```python
from build123d import *

# Parameters (mm, degrees)
SZKIC1_W                                             = 60
SZKIC1_H                                             = 62
DODANIE_WYCI_GNI_CIE1_DEPTH                          = 12
SZKIC2_R                                             = 17
WYTNIJ_WYCI_GNI_CIE1_DEPTH                           = 337.608080711
POG_BIENIE_WALCOWE_POD_M5_WKR_T_DO_CZ_CI_D           = 5.5
POG_BIENIE_WALCOWE_POD_M5_WKR_T_DO_CZ_CI_CBORE_D     = 9
POG_BIENIE_WALCOWE_POD_M5_WKR_T_DO_CZ_CI_CBORE_DEPTH = 5
OTW_R_GWINTOWANY_M5X0_81_D                           = 4.2
SFAZOWANIE1_SIZE                                     = 5


with BuildPart() as part:
    # Szkic1 → Dodanie-wyciągnięcie1 (new body)
    with BuildSketch(Plane.XY):
        with Locations((30, 300)):
            Rectangle(SZKIC1_W, SZKIC1_H)
    extrude(amount=DODANIE_WYCI_GNI_CIE1_DEPTH)

    # Szkic2 → Wytnij-wyciągnięcie1 (cut, through all)
    with BuildSketch(Plane.XY.offset(12)):
        with Locations((31.5, 300)):
            Circle(SZKIC2_R)
    extrude(amount=-WYTNIJ_WYCI_GNI_CIE1_DEPTH, mode=Mode.SUBTRACT)

    # Pogłębienie walcowe pod M5 Wkręt do części metalowych z łbem sześciokątnym1 (through all)
    with Locations(Plane.XY.offset(12)):
        with Locations((6, 314), (6, 286)):
            CounterBoreHole(POG_BIENIE_WALCOWE_POD_M5_WKR_T_DO_CZ_CI_D / 2, POG_BIENIE_WALCOWE_POD_M5_WKR_T_DO_CZ_CI_CBORE_D / 2, POG_BIENIE_WALCOWE_POD_M5_WKR_T_DO_CZ_CI_CBORE_DEPTH)

    # Otwór gwintowany M5x0.81 (through all)
    with Locations(Plane.XY.offset(12)):
        with Locations((55.07, 323.57), (55.07, 276.43), (7.93, 323.57), (7.93, 276.43)):
            Hole(OTW_R_GWINTOWANY_M5X0_81_D / 2)

    # Sfazowanie1
    sfazowanie1_edges = [part.edges().sort_by_distance(p)[0] for p in [
        (60, 331, 6),
        (60, 269, 6),
    ]]
    chamfer(sfazowanie1_edges, length=SFAZOWANIE1_SIZE)


solid = part.part
```
CAD build for the part. Positions are in the model's coordinates, mm. A direction names the side the tool comes from. Give positions to 0.01 mm unless a question says otherwise; leave off trailing zeros. Loops run counter-clockwise (first coordinate to the right, second up) from the corner with the lowest first, then second, coordinate; pieces in that order, holes last. Notation, with made-up numbers: (-37, 52) - (-33, 52) arc R20 cw to (-33, 56) - close; hole circle Ø4 at (-28.5, 42.5). An arc over 180 degrees is marked (long way). Put each result on its own line as item: value.
Q1. Slice it at D-D (x = 7.93). Give the cut face in (y, z), plus the area to 3 significant figures.
Filled in:
outline: (269, 0) - (274.33, 0) - (274.33, 12) - (269, 12) - close; (278.53, 0) - (284.04, 0) - (284.04, 7) - (281.93, 7) - (281.93, 12) - (278.53, 12) - close; (287.96, 0) - (312.04, 0) - (312.04, 7) - (309.93, 7) - (309.93, 12) - (290.07, 12) - (290.07, 7) - (287.96, 7) - close; (315.96, 0) - (321.47, 0) - (321.47, 12) - (318.07, 12) - (318.07, 7) - (315.96, 7) - close; (325.67, 0) - (331, 0) - (331, 12) - (325.67, 12) - close
area: 507 mm²
Q2. Flat gauge pin, fed straight in: pin 1 (7 mm diameter, centred on x = 6, y = 314, fed in from +Z). Where does the tip first touch, or does it go through?
Filled in:
pin 1: stops at z = 7
Q3. Tool access for faces 1 (the face through (5.02, 309.61, 9.54)), 2 (the face through (16, 314, 0)): list every direction of +Z, -Z, +X, -X, +Y, -Y with a clear straight run to the whole face (end or side of a thin tool).
Filled in:
face 1: +Z
face 2: -Z, +X, -X, +Y, -Y
Q4. Slice it at B-B (y = 276.43). Give the cut face in (x, z).
Filled in:
outline: (0, 0) - (5.83, 0) - (5.83, 12) - (0, 12) - close; (10.03, 0) - (52.97, 0) - (52.97, 12) - (10.03, 12) - close; (57.17, 0) - (60, 0) - (60, 12) - (57.17, 12) - close
Q5. Probe line 1 along X through (y, z) = (276.43, 3); line 2 along X through (y, z) = (278, 1); line 3 along Y through (x, z) = (6.5, 10). List the from-to ranges inside material, lowest first.
Filled in:
line 1: x = 0 to 5.83, 10.03 to 52.97, 57.17 to 60
line 2: x = 0 to 6.54, 9.32 to 53.68, 56.46 to 60
line 3: y = 269 to 274.89, 277.97 to 281.53, 290.47 to 309.53, 318.47 to 322.03, 325.11 to 331
Q6. Mould opens along X. For faces 3 (the face through (6.8, 278.2, 5.9)), 4 (the face through (27, 331, 6)), 5 (the face through (58, 328, 6)) say: pulls with the +X half, pulls with the -X half, needs draft (parallel to the pull), parting line crosses it, or undercut.
Filled in:
face 3: undercut
face 4: needs draft
face 5: pulls with the +X half
Q7. Slice it at C-C (x = 31.5). Give the cut face in (y, z), plus the area to 3 significant figures.
Filled in:
outline: (269, 0) - (283, 0) - (283, 12) - (269, 12) - close; (317, 0) - (331, 0) - (331, 12) - (317, 12) - close
area: 336 mm²
Q8. Slice it at A-A (z = 8). Give the cut face in (x, y), plus the area to 3 significant figures.
Filled in:
outline: (0, 269) - (55, 269) - (60, 274) - (60, 326) - (55, 331) - (0, 331) - close; hole circle Ø9 at (6, 286); hole circle Ø9 at (6, 314); hole circle Ø4.2 at (7.93, 276.43); hole circle Ø4.2 at (7.93, 323.57); hole circle Ø34 at (31.5, 300); hole circle Ø4.2 at (55.07, 276.43); hole circle Ø4.2 at (55.07, 323.57)
area: 2,600 mm²
